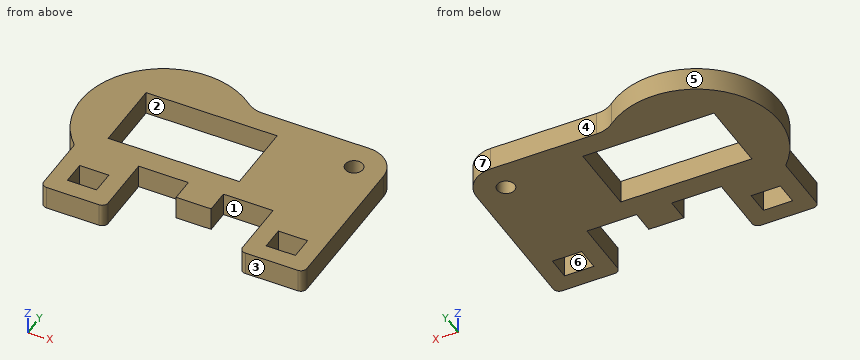
from build123d import *

# Parameters (mm, degrees)
SKETCH1_W           = 22.42
SKETCH1_H           = 12.4
SKETCH1_W_2         = 5
SKETCH1_H_2         = 4
SKETCH1_R           = 1.5
BOSS_EXTRUDE2_DEPTH = 4
FILLET2_R           = 1
FILLET1_R           = 5


with BuildPart() as part:
    # Sketch1 → Boss-Extrude2 (new body)
    with BuildSketch(Plane.XY):
        with BuildLine():
            Line((0, 0), (0, -11))
            Line((0, -11), (11, -11))
            Line((11, -11), (11, 0))
            Line((11, 0), (19.5, 0))
            Line((19.5, 0), (19.5, -4))
            Line((19.5, -4), (25.5, -4))
            Line((25.5, -4), (25.5, 0))
            Line((25.5, 0), (34, 0))
            Line((34, 0), (34, -11))
            Line((34, -11), (45, -11))
            Line((45, -11), (45, 20))
            Line((45, 20), (20, 20))
            ThreePointArc((20, 20), (0, 20), (0, 0))
        make_face()
        with Locations((15.01, 10)):
            Rectangle(SKETCH1_W, SKETCH1_H, mode=Mode.SUBTRACT)
        with Locations((5.5, -6)):
            Rectangle(SKETCH1_W_2, SKETCH1_H_2, mode=Mode.SUBTRACT)
        with Locations((40, 15)):
            Circle(SKETCH1_R, mode=Mode.SUBTRACT)
        with Locations((39.5, -6)):
            Rectangle(SKETCH1_W_2, SKETCH1_H_2, mode=Mode.SUBTRACT)
    extrude(amount=BOSS_EXTRUDE2_DEPTH)

    # Fillet2
    fillet2_edges = [part.edges().sort_by_distance(p)[0] for p in [
        (45, -11, 2),
        (34, -11, 2),
        (11, -11, 2),
        (0, -11, 2),
    ]]
    fillet(fillet2_edges, radius=FILLET2_R)

    # Fillet1
    fillet1_edges = [part.edges().sort_by_distance(p)[0] for p in [
        (45, 20, 2),
        (20, 20, 2),
    ]]
    fillet(fillet1_edges, radius=FILLET1_R)


solid = part.part
Read the model definition and answer for the solid it produces. Units are mm, in the model's axes. Face numbers are marked on the shaded views. A direction names the side the tool comes from. Coordinates: 2 decimals unless noted, no trailing zeros. Order: outer loops, then holes, each group sorted by start corner. A loop starts at its lowest first (then second) coordinate and runs counter-clockwise, first axis right, second up. Notation, with made-up numbers: M 31,57 L 68,57 A31 ccw 68,93 Z; hole C 4.25,32 d7. An arc over 180 degrees is marked long. Put each result on its own line as item: value. Start each with the question number.
Item 1: Given pin 1 Ø1.2 at (x, z) = (31.5, 2) entering from -Y; pin 2 Ø1.2 at (x, z) = (34.5, 2.5) entering from +Y; pin 3 Ø2 at (x, z) = (24, 1.5) entering from -Y, each flat-ended and moving along its own axis, determine where each tip first touches the part or whether it passes through.
Item 2: Consider probe 1 along Y at (x, z) = (40, 1.1); probe 2 along X at (y, z) = (-4.5, 2.3); probe 3 along X at (y, z) = (-0.5, 1.4). Determine where each line is inside the solid, lowest interval first. Write a range as [from, to].
Item 3: Section C-C, the plane z = 1.6 is taken. Count the separate pieces of the cut face and the enclosed holes in it, plus the area to 3 significant figures.
Item 4: The mould has two halves that part along X. Classify the marked faces 5, 6 and 7: +X half, -X half, draft (parallel to the pull), parting line (faces both ways), or undercut.
Item 5: For the marked faces 1, 2, 3 and 4, determine the directions among +Z, -Z, +X, -X, +Y, -Y from which every point of the face is accessible in a straight line to the end or side of a thin tool.
Item 6: Section A-A, the plane x = 25 is taken. Determine the outline of the cut face in (y, z), plus the area to 3 significant figures.
Item 7: Section D-D, the plane x = 36.5 is taken. Determine the outline of the cut face in (y, z), plus the area to 3 significant figures.
Item 8: Section B-B, the plane y = 10 is taken. Determine the outline of the cut face in (x, z), plus the area to 3 significant figures.
Computed:
1. pin 1: stops at y = 0
1. pin 2: stops at y = 20
1. pin 3: stops at y = -4
2. probe 1: y = [-11, -8], [-4, 13.5], [16.5, 20]
2. probe 2: x = [0, 3], [8, 11], [34, 37], [42, 45]
2. probe 3: x = [0, 11], [19.5, 25.5], [34, 45]
3. separate pieces: 1
3. enclosed holes: 4
3. area: 949 mm2
4. face 5: parting line
4. face 6: undercut
4. face 7: +X half
5. face 1: +Z, -Z, -Y
5. face 2: +Z, -Z
5. face 3: +Z, -Z, +X, -X, -Y
5. face 4: +Z, -Z, +X, +Y
6. outline: M -4,0 L 3.8,0 L 3.8,4 L -4,4 Z; M 16.2,0 L 20,0 L 20,4 L 16.2,4 Z
6. area: 46.4 mm2
7. outline: M -11,0 L 20,0 L 20,4 L -11,4 Z
7. area: 124 mm2
8. outline: M -4.14,0 L 3.8,0 L 3.8,4 L -4.14,4 Z; M 26.22,0 L 45,0 L 45,4 L 26.22,4 Z
8. area: 107 mm2
